Source: three-view drawing plus pictorial views. Frame: mm from the lowest corner of the part. Give positions to 0.01 mm unless a question says otherwise; leave off trailing zeros. Loops run counter-clockwise (first coordinate to the right, second up) from the corner with the lowest first, then second, coordinate; pieces in that order, holes last. Notation, with made-up numbers: M 79,-39.5 L 120,-39.5 A24 ccw 120,-25.5 Z; hole C 75.25,24.5 d4. An arc over 180 degrees is marked long. Answer as a JSON object with one key per item and string values. Group by question number.
1) First-contact query: P1, Ø2, axis at y = 0.5, z = 2, coming from the -X side. Flat tip, straight axial feed; report the tip coordinate or a pass-through.
2) Section query B-B on z = 5. Return loops of the section in (x, y) (1 decimal).
3) Ray query, L1, parallel to X at y = 1.05, z = 4; L2, parallel to X at y = 3.6, z = 3 (1 decimal); L3, parallel to Z at x = 91, y = 2.05. Return the intervals inside material, ascending.
4) Section query A-A on y = 1.75. Count the separate pieces of the cut face and the enclosed holes in it, plus the area to 3 significant figures.
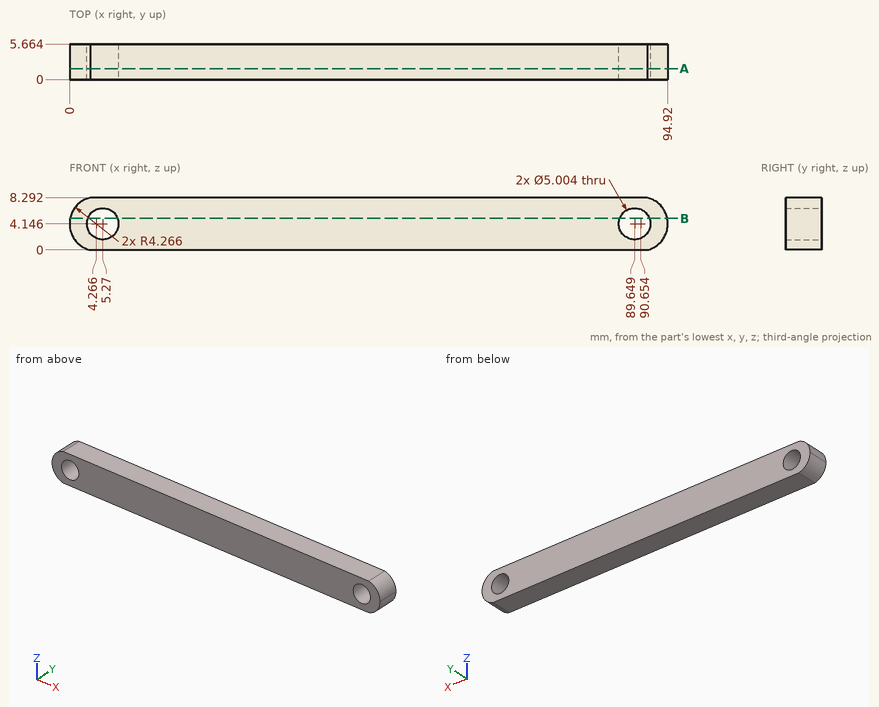
Output:
{
 "1": {"P1": "stops at x = 0.16"},
 "2": {"outline": "M 0.1,0 L 2.9,0 L 2.9,5.7 L 0.1,5.7 Z; M 7.6,0 L 87.3,0 L 87.3,5.7 L 7.6,5.7 Z; M 92,0 L 94.8,0 L 94.8,5.7 L 92,5.7 Z"},
 "3": {"L1": "x = 0 to 2.77, 7.77 to 87.15, 92.15 to 94.92", "L2": "x = 0.2 to 3, 7.5 to 87.4, 91.9 to 94.8", "L3": "z = 0 to 2.04, 6.25 to 8.29"},
 "4": {"separate pieces": "1", "enclosed holes": "2", "area": "734 mm^2"}
}
